Work out the finished part from the listing and answer in its coordinate system (mm). Coordinates: 2 decimals unless noted, no trailing zeros. Order: outer loops, then holes, each group sorted by start corner. A loop starts at its lowest first (then second) coordinate and runs counter-clockwise, first axis right, second up.
```python
from build123d import *

# Parameters (mm, degrees)
SKETCH1_R               = 394.45
SKETCH1_R_2             = 337.3
BOSS_EXTRUDE1_DEPTH     = 9.525
SKETCH2_W               = 63.5
SKETCH2_H               = 206.256826312
CUT_EXTRUDE1_DEPTH      = 10.525
BOSS_EXTRUDE4_DEPTH     = 9.525
F_3_8_CLEARANCE_HOLE1_D = 10.31748
MIRROR3_COPY_1_D        = 10.31748
F_3_8_CLEARANCE_HOLE2_D = 10.31748
CIRPATTERN1_COUNT       = 8
CUT_EXTRUDE5_DEPTH      = 10.525
MIRROR9_COPY_1_DEPTH    = 10.525


with BuildPart() as part:
    # Sketch1 → Boss-Extrude1 (new body)
    with BuildSketch(Plane(origin=(0, 0, 0), x_dir=(1, 0, 0), z_dir=(0, 1, 0))):
        Circle(SKETCH1_R)
        Circle(SKETCH1_R_2, mode=Mode.SUBTRACT)
    extrude(amount=BOSS_EXTRUDE1_DEPTH)

    # Sketch2 → Cut-Extrude1 (cut, through all)
    with BuildSketch(Plane(origin=(0, 9.525, 0), x_dir=(1, 0, 0), z_dir=(0, 1, 0))):
        with Locations((-412.48, 0)):
            Rectangle(SKETCH2_W, SKETCH2_H)
    extrude(amount=-CUT_EXTRUDE1_DEPTH, mode=Mode.SUBTRACT)

    # Sketch5 → Boss-Extrude4 (add)
    with BuildSketch(Plane(origin=(0, 0, 0), x_dir=(1, 0, 0), z_dir=(0, 1, 0))):
        with BuildLine():
            Line((278.064904497, 190.921970677), (417.548677299, 190.921970677))
            Line((417.548677299, 190.921970677), (417.548677299, -190.921970677))
            Line((417.548677299, -190.921970677), (278.064904497, -190.921970677))
            ThreePointArc((278.064904497, -190.921970677), (337.3, 0), (278.064904497, 190.921970677))
        make_face()
    boss_extrude4 = extrude(amount=BOSS_EXTRUDE4_DEPTH)

    # Mirror1: Boss-Extrude4 across plane
    add(boss_extrude4.mirror(Plane(origin=(0, 0, 0), x_dir=(0, 0, 1), z_dir=(1, 0, 0))))

    # 3/8 Clearance Hole1 (through all)
    with Locations(Plane(origin=(0, 9.525, 0), x_dir=(-1, 0, 0), z_dir=(0, 1, 0))):
        with Locations((-329.955744274, 116.744193948), (-309.58033967, 163.278943192)):
            f_3_8_clearance_hole1 = Hole(F_3_8_CLEARANCE_HOLE1_D / 2)

    # Mirror2: 3/8 Clearance Hole1 across plane
    add(f_3_8_clearance_hole1.mirror(Plane(origin=(0, 0, 0), x_dir=(0, 0, 1), z_dir=(1, 0, 0))), mode=Mode.SUBTRACT)

    # Mirror3: 3/8 Clearance Hole1 across plane
    add(f_3_8_clearance_hole1.mirror(Plane.XY), mode=Mode.SUBTRACT)

    # Mirror3 copy 1 (through all)
    with Locations(Plane(origin=(0, 9.525, 0), x_dir=(1, 0, 0), z_dir=(0, 1, 0))):
        with Locations((-329.955744274, 116.744193948), (-309.58033967, 163.278943192)):
            Hole(MIRROR3_COPY_1_D / 2)

    # 3/8 Clearance Hole2 (through all)
    with Locations(Plane(origin=(0, 9.525, 0), x_dir=(1, 0, 0), z_dir=(0, 1, 0))):
        with Locations((247.487373415, -247.487373415)):
            f_3_8_clearance_hole2 = Hole(F_3_8_CLEARANCE_HOLE2_D / 2)

    # CirPattern1: 3/8 Clearance Hole2 ×8 about axis, 2 skipped
    cirpattern1_axis = Axis((0, 0, 0), (0, 1, 0))
    add([f_3_8_clearance_hole2.rotate(cirpattern1_axis, i * 360 / CIRPATTERN1_COUNT) for i in range(1, CIRPATTERN1_COUNT) if i not in (1, 5)], mode=Mode.SUBTRACT)

    # Sketch12 → Cut-Extrude5 (cut, through all)
    with BuildSketch(Plane(origin=(0, 0, 0), x_dir=(1, 0, 0), z_dir=(0, 1, 0))):
        Polygon((-417.548677299, 190.921970677), (-417.548677299, 73.2544087), (-345.166052231, 190.921970677), align=None)
    cut_extrude5 = extrude(amount=CUT_EXTRUDE5_DEPTH, mode=Mode.SUBTRACT)

    # Mirror8: Cut-Extrude5 across plane
    add(cut_extrude5.mirror(Plane.XY), mode=Mode.SUBTRACT)

    # Mirror9: Cut-Extrude5 across plane
    add(cut_extrude5.mirror(Plane(origin=(0, 0, 0), x_dir=(0, 0, 1), z_dir=(1, 0, 0))), mode=Mode.SUBTRACT)

    # Mirror9 copy 1 sketch → Mirror9 copy 1 (cut, through all)
    with BuildSketch(Plane(origin=(0, 0, 0), x_dir=(-1, 0, 0), z_dir=(0, 1, 0))):
        Polygon((-417.548677299, 190.921970677), (-417.548677299, 73.2544087), (-345.166052231, 190.921970677), align=None)
    extrude(amount=MIRROR9_COPY_1_DEPTH, mode=Mode.SUBTRACT)


solid = part.part
```
1. The part is cut by section C-C (y = 5.75). Count the separate pieces of the cut face and the enclosed holes in it, plus the area to 3 significant figures.
2. The part is cut by section B-B (x = 230). Determine the outline of the cut face in (y, z) (3 decimals).
3. Consider probe 1 along Z at (x, y) = (0, 7.75); probe 2 along X at (y, z) = (1, -118.5) (1 decimal); probe 3 along X at (y, z) = (4.5, 235). Determine where each line is inside the solid, lowest interval first.
4. Flat-ended cylindrical pins translate along their axes: pin 1 (12 mm diameter, centred on x = 309.58, z = -163.28, fed in from +Y) (3 decimals); pin 2 (8.5 mm diameter, centred on x = 329.96, z = 116.74, fed in from +Y); pin 3 (1.5 mm diameter, centred on x = 196.5, y = 7.5, fed in from -Z); pin 4 (1 mm diameter, centred on x = -185.5, y = 7.5, fed in from +Z). Find the tip coordinate at first contact, or state that the pin passes through.
5. The part is cut by section A-A (z = 0). Determine the outline of the cut face in (x, y) (3 decimals), plus the area to 3 significant figures.
Worked out:
1. separate pieces: 1
1. enclosed holes: 15
1. area: 143,000 mm2
2. outline: (0, -320.454) - (9.525, -320.454) - (9.525, -246.721) - (0, -246.721) - close; (0, 246.721) - (9.525, 246.721) - (9.525, 320.454) - (0, 320.454) - close
3. probe 1: z = -394.45 to -355.16, -344.84 to -337.3, 337.3 to 344.84, 355.16 to 394.45
3. probe 2: x = -389.7 to -334.8, -325.1 to -315.8, 315.8 to 325.1, 334.8 to 389.7
3. probe 3: x = -316.81 to -241.96, 241.96 to 316.81
4. pin 1: stops at y = 9.525
4. pin 2: passes through
4. pin 3: stops at z = -342.45
4. pin 4: stops at z = 348.38
5. outline: (-417.549, 0) - (-337.3, 0) - (-337.3, 9.525) - (-417.549, 9.525) - close; (337.3, 0) - (417.549, 0) - (417.549, 9.525) - (337.3, 9.525) - close
5. area: 1,530 mm2
